Design review of the part built by this model. Coordinates are the model's own, in mm. A direction names the side the tool comes from. Coordinates: 2 decimals unless noted, no trailing zeros. Loops run counter-clockwise (first coordinate to the right, second up) from the corner with the lowest first, then second, coordinate; pieces in that order, holes last. Notation, with made-up numbers: (-34, 36) - (-1, 36) arc R16 cw to (-1, 55) - close; hole circle Ø4 at (80, -40). An arc over 180 degrees is marked (long way). Use one line per item in the form item = value. Start each with the question number.
(1) Tool access review of faces 4 (the face through (-11, -5, 0)), 5 (the face through (9, 13, 0)), 6 (the face through (0, 9.5, 0)), 7 (the face through (-5, -11, 0)), 8 (the face through (11, -5, 0)): name each direction out of +Z, -Z, +X, -X, +Y, -Y from which nothing blocks a thin tool from reaching the whole face with its end or side.
(2) For L1, parallel to Y at x = -10.25, z = -0.1; L2, parallel to Y at x = 3, z = -1.6, list the stretches that pass through material, from the lowest coordinate up.
(3) Clearance check with flat-ended pins moving along their axes: pin 1 Ø2 at (y, z) = (0, -1.5) entering from -X; pin 2 Ø1.8 at (x, z) = (0.5, -1) entering from +Y; pin 3 Ø2 at (x, z) = (-2.5, -0.5) entering from -Y. State where each tip first meets the part, or that it passes through.
(4) Add section B-B (z = -1.1). State the section outline as (x, y) points.
(5) Add section A-A (y = 11.25). State the section outline as (x, z) points, plus the area to 3 significant figures.
(6) The part is to be moulded in two halves that separate along Y. For faces 1 (the face through (-13, -9, 0)), 2 (the face through (-11, 5, 0)), 3 (the face through (-9, -13, 0)), say which applies: pulls with the +Y half, pulls with the -Y half, needs draft (parallel to the pull), parting line crosses it, or undercut.
(7) Add section C-C (x = 4.5). State the section outline as (y, z) points, plus the area to 3 significant figures.
Autodesk Inventor part; units mm, degrees
ref_plane "YZ Plane" through (0, 0, 0) normal (1, 0, 0) x (0, 1, 0)
ref_plane "XZ Plane" through (0, 0, 0) normal (0, 1, 0) x (-1, 0, 0)
ref_plane "XY Plane" through (0, 0, 0) normal (0, 0, 1) x (1, 0, 0)
sketch "Sketch1" plane through (0, 0, 0) normal (0, 0, 1) x (1, 0, 0)
  circle A0 centre (0, 0) radius 6
  line L0 (-13, 13) -> (13, 13)
  line L1 (13, 13) -> (13, -13)
  line L2 (13, -13) -> (-13, -13)
  line L3 (-13, -13) -> (-13, 13)
  line L4 (0, 0) -> (13, 13)
  line L5 (6.5, 6.5) -> (13, 13)
  circle A1 centre (9.75, 9.75) radius 0.5
  line L6 (0, 0) -> (-13, 13)
  line L7 (-6.5, 6.5) -> (-13, 13)
  circle A2 centre (-9.75, 9.75) radius 0.5
  line L8 (0, 0) -> (-13, -13)
  line L9 (-6.5, -6.5) -> (-13, -13)
  circle A3 centre (-9.75, -9.75) radius 0.5
  line L10 (0, 0) -> (13, -13)
  line L11 (6.5, -6.5) -> (13, -13)
  circle A4 centre (9.75, -9.75) radius 0.5
  line L12 (-5, -13) -> (5, -13)
  line L13 (5, -13) -> (5, -9.5)
  line L14 (5, -9.5) -> (-5, -9.5)
  line L15 (-5, -9.5) -> (-5, -13)
  line L16 (13, 5) -> (9.5, 5)
  line L17 (9.5, 5) -> (9.5, -5)
  line L18 (9.5, -5) -> (13, -5)
  line L19 (-5, 13) -> (-5, 9.5)
  line L20 (-5, 9.5) -> (5, 9.5)
  line L21 (5, 9.5) -> (5, 13)
  line L22 (-13, -5) -> (-9.5, -5)
  line L23 (-9.5, -5) -> (-9.5, 5)
  line L24 (-9.5, 5) -> (-13, 5)
  point P0 (0, 13)
  point P1 (13, 0)
  point P2 (0, -9.5)
  point P3 (0, -13)
  point P4 (9.5, 0)
  point P5 (0, 9.5)
  point P6 (-9.5, 0)
  dimension "d4" = 12
  dimension "d5" = 26
  dimension "d6" = 26
  dimension "d7" = 1
  dimension "d8" = 360
  dimension "d9" = 10
  dimension "d10" = 3.5
  dimension "d11" = 360
extrude "Extrusion1" add sketch "Sketch1" along normal mid plane 3.5 contours A0 L10 L4 | A0 L4 A1 L1 L16 L17 L18 L10 A4 | L4 L6 A0 | A0 L6 A2 L0 L19 L20 L21 L4 A1 | L10 A4 L2 L13 L14 L15 L8 A3 A0 | A0 L8 L10 | L6 L8 A0 | A0 L8 A3 L3 L22 L23 L24 L6 A2 | A1 L4 | L4 A1 | A4 L10 | L10 A4 | A2 L6 | L6 A2 | A3 L8 | L8 A3
equation "\"d6\" = d5"
properties part number "Spodi Spodnji"
Computed values:
q1.face_4 = +Z, -Z, -X
q1.face_5 = +Z, -Z, +X, -X, +Y
q1.face_6 = +Z, -Z, +Y
q1.face_7 = +Z, -Z, -Y
q1.face_8 = +Z, -Z, +X
q2.L1 = -13 to -5, 5 to 13
q2.L2 = -9.5 to 9.5
q3.pin_1 = -9.5
q3.pin_2 = 9.5
q3.pin_3 = -9.5
q4.outline = (-13, -13) - (-5, -13) - (-5, -9.5) - (5, -9.5) - (5, -13) - (13, -13) - (13, -5) - (9.5, -5) - (9.5, 5) - (13, 5) - (13, 13) - (5, 13) - (5, 9.5) - (-5, 9.5) - (-5, 13) - (-13, 13) - (-13, 5) - (-9.5, 5) - (-9.5, -5) - (-13, -5) - close
q5.outline = (-13, -1.75) - (-5, -1.75) - (-5, 1.75) - (-13, 1.75) - close; (5, -1.75) - (13, -1.75) - (13, 1.75) - (5, 1.75) - close
q5.area = 56.0 mm^2
q6.face_1 = needs draft
q6.face_2 = undercut
q6.face_3 = pulls with the -Y half
q7.outline = (-9.5, -1.75) - (9.5, -1.75) - (9.5, 1.75) - (-9.5, 1.75) - close
q7.area = 66.5 mm^2
